```python
from build123d import *

# Parameters (mm, degrees)
SKETCH_1_R                    = 6
SKETCH_1_R_2                  = 3
EXTRUDE_1_DEPTH               = 50.5
CUT_EXTRUDE_2_DEPTH           = 50.5
CUT_EXTRUDE_2_DEPTH_BACK      = 58.831652233
SKETCH_3_R                    = 3.1
SKETCH_3_W                    = 28.166385617
SKETCH_3_H                    = 19.728727066
SKETCH_3_W_2                  = 28.6736781
SKETCH_3_H_2                  = 13.5
CUT_EXTRUDE_START             = 6.5
CUT_EXTRUDE_3_DEPTH           = 50.5
CHAMFER_1_SIZE                = 3
CUT_EXTRUDE_START_2           = 2.5
SKETCH_3_2_R                  = 3.1
CUT_EXTRUDE_5_DEPTH           = 10
CUT_EXTRUDE_5_DRAFT           = -40
CUT_EXTRUDE_5_PROFILE_2_DEPTH = 10
CUT_EXTRUDE_5_PROFILE_2_DRAFT = -40


with BuildPart() as part:
    # Sketch 1 → Extrude 1 (new body)
    # profile 1 of 2: a face of its own
    with BuildSketch(Plane.XY):
        with BuildLine():
            Line((0, 0), (25.5, 0))
            Line((25.5, 0), (25.5, 6))
            Line((25.5, 6), (6, 6))
            ThreePointArc((6, 6), (4.242640687, 1.757359313), (0, 0))
        make_face()
    # profile 2 of 2: a face of its own
    with BuildSketch(Plane.XY):
        with Locations((0, 6)):
            Circle(SKETCH_1_R)
        with Locations((0, 6)):
            Circle(SKETCH_1_R_2, mode=Mode.SUBTRACT)
    extrude(amount=EXTRUDE_1_DEPTH)

    # Sketch 3 → Cut-Extrude 2 (cut, two sides: drawn at the far end of the back side and taken through both)
    with BuildSketch(Plane(origin=(0, 0, 0), x_dir=(1, 0, 0), z_dir=(0, 1, 0)).offset(-CUT_EXTRUDE_2_DEPTH_BACK)):
        with Locations(Location((15.5, -9.75, 0), (0, 0, 270))):
            Circle(SKETCH_3_R)
        with Locations(Location((15.5, -40.75, 0), (0, 0, 270))):
            Circle(SKETCH_3_R)
        with Locations((-8.083192809, -48.364363533)):
            Rectangle(SKETCH_3_W, SKETCH_3_H)
        with Locations((-8.33683905, -18.75)):
            Rectangle(SKETCH_3_W_2, SKETCH_3_H_2)
    extrude(amount=CUT_EXTRUDE_2_DEPTH + CUT_EXTRUDE_2_DEPTH_BACK, mode=Mode.SUBTRACT)

    # Sketch 4 → Cut-Extrude 3 (cut)
    with BuildSketch(Plane(origin=(0, 0, 0), x_dir=(0, 0, -1), z_dir=(1, 0, 0)).offset(CUT_EXTRUDE_START)):
        Polygon((0, 6), (-3, 6), (0, 3), align=None)
    extrude(amount=CUT_EXTRUDE_3_DEPTH, mode=Mode.SUBTRACT)

    # Chamfer 1
    chamfer_1_edges = [part.edges().sort_by_distance(p)[0] for p in [
        (15.75, 6, 50.5),
        (25.5, 6, 26.75),
    ]]
    chamfer(chamfer_1_edges, length=CHAMFER_1_SIZE)


with BuildPart() as cut_extrude_5_tool:
    # Sketch 3_2 → Cut-Extrude 5 (with draft: the straight prism first)
    with BuildSketch(Plane(origin=(0, 0, 0), x_dir=(1, 0, 0), z_dir=(0, 1, 0)).offset(CUT_EXTRUDE_START_2)):
        with Locations(Location((15.5, -9.75, 0), (0, 0, 270))):
            Circle(SKETCH_3_2_R)
    extrude(amount=CUT_EXTRUDE_5_DEPTH)
    # Cut-Extrude 5: the draft: its side faces are tilted about the plane it starts from
    cut_extrude_5_sides = [cut_extrude_5_tool.faces().sort_by_distance(p)[0] for p in [
        (15.5, 7.5, 6.65),
    ]]
    draft(cut_extrude_5_sides, Plane(origin=(0, 0, 0), x_dir=(1, 0, 0), z_dir=(0, 1, 0)).offset(CUT_EXTRUDE_START_2), CUT_EXTRUDE_5_DRAFT)


with BuildPart() as part_1:
    add(part.part)

    # Cut-Extrude 5: cut by cut_extrude_5_tool
    add(cut_extrude_5_tool.part, mode=Mode.SUBTRACT)


with BuildPart() as cut_extrude_5_profile_2_tool:
    # Sketch 3_2 → Cut-Extrude 5 profile 2 (with draft: the straight prism first)
    with BuildSketch(Plane(origin=(0, 0, 0), x_dir=(1, 0, 0), z_dir=(0, 1, 0)).offset(CUT_EXTRUDE_START_2)):
        with Locations(Location((15.5, -40.75, 0), (0, 0, 270))):
            Circle(SKETCH_3_2_R)
    extrude(amount=CUT_EXTRUDE_5_PROFILE_2_DEPTH)
    # Cut-Extrude 5 profile 2: the draft: its side faces are tilted about the plane it starts from
    cut_extrude_5_profile_2_sides = [cut_extrude_5_profile_2_tool.faces().sort_by_distance(p)[0] for p in [
        (15.5, 7.5, 37.65),
    ]]
    draft(cut_extrude_5_profile_2_sides, Plane(origin=(0, 0, 0), x_dir=(1, 0, 0), z_dir=(0, 1, 0)).offset(CUT_EXTRUDE_START_2), CUT_EXTRUDE_5_PROFILE_2_DRAFT)


with BuildPart() as part_2:
    add(part_1.part)

    # Cut-Extrude 5 profile 2: cut by cut_extrude_5_profile_2_tool
    add(cut_extrude_5_profile_2_tool.part, mode=Mode.SUBTRACT)


solid = part_2.part
```
Source: CAD feature listing. Evaluate the final solid. Frame: model axes, mm. A direction names the side the tool comes from. Round coordinates to 2 decimals unless told otherwise and drop trailing zeros. Loops run counter-clockwise (first coordinate to the right, second up) from the corner with the lowest first, then second, coordinate; pieces in that order, holes last.
(1) Access query for faces 1 (the flat face through (6, 3, 45)), 2 (the flat face through (16, 5, 2)), 3 (the conical face through (18.715, 2.67, 40.328)), 4 (the flat face through (1, 3, 12)), 5 (the flat face through (15.9, 4.5, 49)). Directions: +Z, -Z, +X, -X, +Y, -Y. A direction counts if a zero-diameter tool reaches every point of the face in a straight line with its end or side. Return the directions, or none.
From the geometry:
face 1: +Z, -X, +Y, -Y
face 2: -Z, +X, +Y
face 3: +Y
face 4: -X, +Y, -Y
face 5: +Z, +X, -X, +Y
(2) Section query B-B (x = 15.5). Output: boundary loops of the cut face in (y, z).
From the geometry:
outline: (0, 0) - (3, 0) - (6, 3) - (6, 3.71) - (2.5, 6.65) - (0, 6.65) - close; (0, 12.85) - (2.5, 12.85) - (6, 15.79) - (6, 34.71) - (2.5, 37.65) - (0, 37.65) - close; (0, 43.85) - (2.5, 43.85) - (6, 46.79) - (6, 47.5) - (3, 50.5) - (0, 50.5) - close
(3) Section query A-A (y = 4). Output: boundary loops of the cut face in (x, z), and give its area (3 significant figures).
From the geometry:
outline: (-5.66, 0) - (-2.24, 0) - (-2.24, 12) - (-5.66, 12) - close; (-5.66, 25.5) - (-2.24, 25.5) - (-2.24, 38.5) - (-5.66, 38.5) - close; (2.24, 0) - (6.5, 0) - (6.5, 1) - (24.5, 1) - (24.5, 49.5) - (6, 49.5) - (6, 38.5) - (2.24, 38.5) - (2.24, 25.5) - (6, 25.5) - (6, 12) - (2.24, 12) - close; hole circle Ø8.72 at (15.5, 9.75); hole circle Ø8.72 at (15.5, 40.75)
area: 958 mm2
(4) Material intervals for probe 1 along Z at (x, y) = (15.5, 1.05); probe 2 along Y at (x, z) = (0, 30.5); probe 3 along X at (y, z) = (1.1, 40.75), sorted ascending.
From the geometry:
probe 1: z = 0 to 6.65, 12.85 to 37.65, 43.85 to 50.5
probe 2: y = 0 to 3, 9 to 12
probe 3: x = 6 to 12.4, 18.6 to 25.5
(5) Contact query for flat-ended pins moving along their axis: pin 1 Ø8.5 at (x, z) = (13.5, 13) entering from +Y; pin 2 Ø5 at (y, z) = (2, 16.5) entering from -X; pin 3 Ø2.5 at (y, z) = (5, 1) entering from +X; pin 4 Ø3.5 at (x, z) = (15.5, 40.75) entering from +Y. Output: stop coordinate, or through.
From the geometry:
pin 1: stops at y = 6
pin 2: stops at x = 6
pin 3: stops at x = 24.75
pin 4: passes through
(6) Pull-direction query (Z, two-part tool) for faces 6 (the flat face through (16, 2, 50.5)), 7 (the flat face through (6, 3, 19)), 8 (the flat face through (14, 6, 29)); classes: +Z half, -Z half, draft (parallel to the pull), parting line (faces both ways), or undercut.
From the geometry:
face 6: +Z half
face 7: undercut
face 8: draft
(7) Section query D-D (x = 8.5). Output: boundary loops of the cut face in (y, z).
From the geometry:
outline: (0, 0) - (3, 0) - (6, 3) - (6, 47.5) - (3, 50.5) - (0, 50.5) - close
(8) Section query C-C (y = 6.75). Output: boundary loops of the cut face in (x, z), and give its area (3 significant figures).
From the geometry:
outline: (-5.95, 0) - (-2.9, 0) - (-2.9, 12) - (-5.95, 12) - close; (-5.95, 25.5) - (-2.9, 25.5) - (-2.9, 38.5) - (-5.95, 38.5) - close; (2.9, 0) - (5.95, 0) - (5.95, 12) - (2.9, 12) - close; (2.9, 25.5) - (5.95, 25.5) - (5.95, 38.5) - (2.9, 38.5) - close
area: 152 mm2
